Can you work these out from the drawing? Everything is in mm from the part's minimum corner. A direction names the side the tool comes from. Coordinates: 2 decimals unless noted, no trailing zeros. Write each loop counter-clockwise with the first axis right and the second up, starting at its lowest first coordinate (ties: lowest second). Pieces come first, ordered by that corner, then holes. Notation, with made-up numbers: (3.5, 46) -> (50.5, 46) arc R9 cw to (50.5, 55) -> close; hole circle Ø6 at (0, 33). An arc over 180 degrees is marked (long way). Use a Markdown table: item, result. Add a question column.
Item 1: Imagine slicing it at B-B, the plane z = 21.5. Write out the boundary of the cut face in (x, y).
Item 2: Imagine slicing it at D-D, the plane x = 19. Write out the boundary of the cut face in (y, z), and give its area (3 significant figures).
Item 3: Imagine slicing it at C-C, the plane y = 14.5. Count the separate pieces of the cut face and the enclosed holes in it, and give its area (3 significant figures).
Item 4: Imagine slicing it at A-A, the plane x = 5. Write out the boundary of the cut face in (y, z).
Item 5: Will this pin go through, and if not, where does the flat tip stop? pin 1 Ø3 at (x, z) = (5, 5) entering from +Y.
Item 6: If I drill on line 1 along Z through (x, y) = (15.5, 35.5); line 2 along Z through (x, y) = (5.5, 34) (1 decimal); line 3 along X through (y, z) = (12, 5), over which ranges is the centre line in solid material (lowest first)? Write a range as from..to.
Item 7: On a 3-axis mill with a long thin cutter (end or side, diameter ignored), from which of +Z, -Z, +X, -X, +Y, -Y can I reach the whole of each face in a straight line? I mean the marked faces 1 and 2. Say none if no direction works.
Item 8: If we mould it in two halves opening along X, with no side actions, what happens to the marked faces 3, 4 and 5? For each: pulls with the +X half, pulls with the -X half, needs draft (parallel to the pull), parting line crosses it, or undercut.
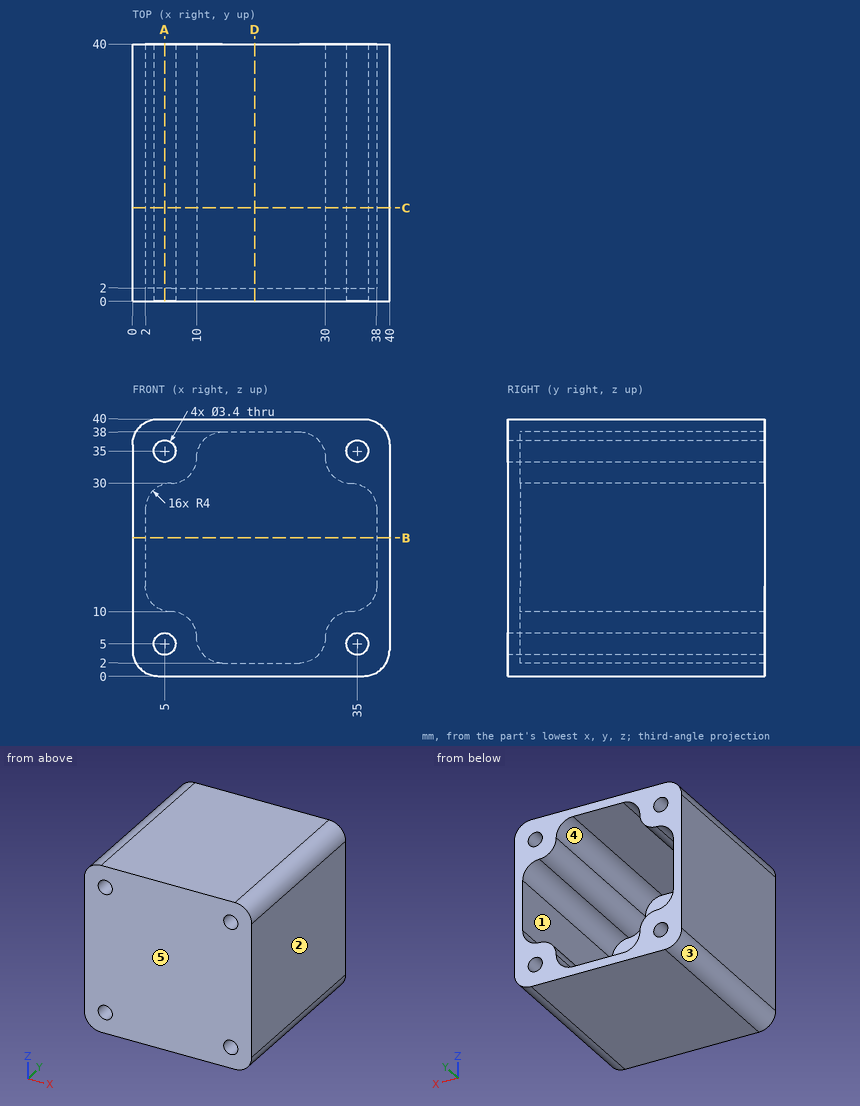
Ans:
| question | item | result |
|---|---|---|
| 1 | outline | (0, 0) -> (40, 0) -> (40, 40) -> (38, 40) -> (38, 2) -> (2, 2) -> (2, 40) -> (0, 40) -> close |
| 2 | outline | (0, 0) -> (40, 0) -> (40, 2) -> (2, 2) -> (2, 38) -> (40, 38) -> (40, 40) -> (0, 40) -> close |
| 2 | area | 232 mm^2 |
| 3 | separate pieces | 1 |
| 3 | enclosed holes | 5 |
| 3 | area | 524 mm^2 |
| 4 | outline | (0, 0) -> (40, 0) -> (40, 3.3) -> (0, 3.3) -> close; (0, 6.7) -> (40, 6.7) -> (40, 10.13) -> (2, 10.13) -> (2, 29.87) -> (40, 29.87) -> (40, 33.3) -> (0, 33.3) -> close; (0, 36.7) -> (40, 36.7) -> (40, 40) -> (0, 40) -> close |
| 5 | pin 1 | passes through |
| 6 | line 1 | z = 0..2, 38..40 |
| 6 | line 2 | z = 0..3.4, 6.6..10, 30..33.4, 36.6..40 |
| 6 | line 3 | x = 0..3.3, 6.7..10.13, 29.87..33.3, 36.7..40 |
| 7 | face 1 | +Y |
| 7 | face 2 | +Z, -Z, +X, +Y, -Y |
| 8 | face 3 | pulls with the -X half |
| 8 | face 4 | undercut |
| 8 | face 5 | needs draft |
